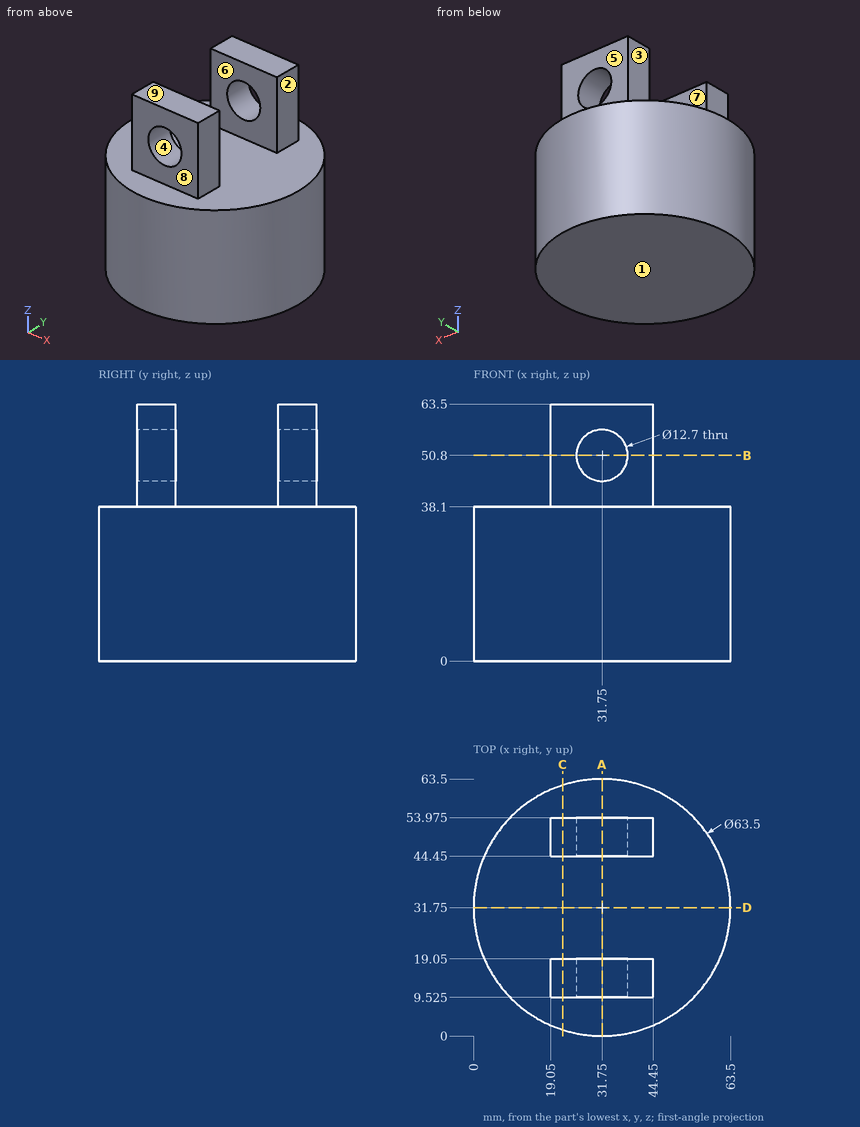
The figure shows three views and two pictorial views of one solid part (mm, origin at its lowest corner). Answer the questions. A direction names the side the tool comes from. Round coordinates to 2 decimals unless told otherwise and drop trailing zeros. Loops run counter-clockwise (first coordinate to the right, second up) from the corner with the lowest first, then second, coordinate; pieces in that order, holes last. Notation, with made-up numbers: (-14.75, -20.5) - (32.25, -20.5) arc R22 cw to (32.25, -9.5) - close; hole circle Ø3 at (-23.5, 15). An arc over 180 degrees is marked (long way). Use one line per item in the form item = value. Start each with the question number.
(1) Find section A-A on x = 31.75. Determine the outline of the cut face in (y, z) (3 decimals).
(2) Which of the six approach directions +Z, -Z, +X, -X, +Y, -Y give full straight-line access (tool end or side, diameter ignored) to the marked faces 1, 2, 3, 4 and 5?
(3) Flat-ended cylindrical pins translate along their axes: P1, Ø20.5, axis at x = 27.5, z = 50.5, coming from the +Y side (3 decimals); P2, Ø20.5, axis at x = 28.5, z = 54, coming from the -Y side (3 decimals); P3, Ø3, axis at x = 50, z = 32, coming from the +Y side. Find the tip coordinate at first contact, or state that the pin passes through.
(4) Find section B-B on z = 50.8. Determine the outline of the cut face in (x, y) (3 decimals), and give its area (3 significant figures).
(5) Find section D-D on y = 31.75. Determine the outline of the cut face in (x, z).
(6) Determine the mould class of the marked faces 6, 7, 8 and 9 for opening direction Y: +Y half, -Y half, draft (parallel to the pull), parting line (faces both ways), or undercut.
(7) Find section C-C on x = 22. Determine the outline of the cut face in (y, z) (3 decimals), and give its area (3 significant figures).
(8) Consider line 1 (Z direction, x = 31.75, y = 51.25); line 2 (Y direction, x = 22, z = 51) (3 decimals); line 3 (X direction, y = 49, z = 50). Determine where each line is inside the solid, lowest interval first.
Answer list:
q1.outline = (0, 0) - (63.5, 0) - (63.5, 38.1) - (53.975, 38.1) - (53.975, 44.45) - (44.45, 44.45) - (44.45, 38.1) - (19.05, 38.1) - (19.05, 44.45) - (9.525, 44.45) - (9.525, 38.1) - (0, 38.1) - close; (9.525, 57.15) - (19.05, 57.15) - (19.05, 63.5) - (9.525, 63.5) - close; (44.45, 57.15) - (53.975, 57.15) - (53.975, 63.5) - (44.45, 63.5) - close
q2.face_1 = -Z, +X, -X, +Y, -Y
q2.face_2 = +Z, +X, +Y, -Y
q2.face_3 = +Z, -X, +Y, -Y
q2.face_4 = +Y, -Y
q2.face_5 = +Z, +X, -X, +Y
q3.P1 = 53.975
q3.P2 = 9.525
q3.P3 = 58.72
q4.outline = (19.05, 9.525) - (25.4, 9.525) - (25.4, 19.05) - (19.05, 19.05) - close; (19.05, 44.45) - (25.4, 44.45) - (25.4, 53.975) - (19.05, 53.975) - close; (38.1, 9.525) - (44.45, 9.525) - (44.45, 19.05) - (38.1, 19.05) - close; (38.1, 44.45) - (44.45, 44.45) - (44.45, 53.975) - (38.1, 53.975) - close
q4.area = 242 mm^2
q5.outline = (0, 0) - (63.5, 0) - (63.5, 38.1) - (0, 38.1) - close
q6.face_6 = undercut
q6.face_7 = undercut
q6.face_8 = -Y half
q6.face_9 = draft
q7.outline = (1.534, 0) - (61.966, 0) - (61.966, 38.1) - (53.975, 38.1) - (53.975, 63.5) - (44.45, 63.5) - (44.45, 38.1) - (19.05, 38.1) - (19.05, 63.5) - (9.525, 63.5) - (9.525, 38.1) - (1.534, 38.1) - close
q7.area = 2,790 mm^2
q8.line_1 = 0 to 44.45, 57.15 to 63.5
q8.line_2 = 9.525 to 19.05, 44.45 to 53.975
q8.line_3 = 19.05 to 25.45, 38.05 to 44.45
